Design review of the part built by this model. Coordinates are the model's own, in mm. A direction names the side the tool comes from. Coordinates: 2 decimals unless noted, no trailing zeros. Write each loop counter-clockwise with the first axis right and the second up, starting at its lowest first coordinate (ties: lowest second). Pieces come first, ordered by that corner, then holes. Notation, with made-up numbers: (-24.5, -22.75) - (0.5, -22.75) arc R9 ccw to (0.5, -8.75) - close; hole circle Ø1 at (75.5, 23). An arc over 180 degrees is marked (long way). Use a Markdown table: item, result.
from build123d import *

# Parameters (mm, degrees)
F3_DEPTH = 50
F4_DEPTH = 50
F5_DEPTH = 50


with BuildPart() as f3:
    # F0 (on Top) → F3 (new body, symmetric)
    with BuildSketch(Plane.XY):
        Polygon((50, -27.040666), (50, 50), (25.545932, 50), (25.545932, -27.040666), (-25.926208, -27.040666), (-25.926208, -8.301959), (-50, -8.301959), (-50, -27.040666), (-50, -50), (-25.926208, -50), (25.545932, -50), (50, -50), align=None)
    extrude(amount=F3_DEPTH, both=True)

    # F1 (on Front) → F4 (intersect, symmetric)
    with BuildSketch(Plane.XZ):
        Polygon((-29.175453, 50), (-50, 50), (-50, -50), (-29.175453, -50), (-29.175453, 20.161899), (-12.334338, -50), (12.334337, -50), (28.463857, 28.938254), (28.463857, -50), (50, -50), (50, 50), (28.463857, 50), (12.334337, -10.199549), (12.334337, 50), (-12.334338, 50), (-12.334338, -10.436747), align=None)
    extrude(amount=F4_DEPTH, both=True, mode=Mode.INTERSECT)

    # F2 (on Right) → F5 (intersect, symmetric)
    with BuildSketch(Plane.YZ):
        Polygon((-26.566265, 50), (-50, 50), (-50, -50), (-26.566265, -50), (-26.566265, 27.98946), (-9.725152, -50), (11.148345, -50), (27.752262, 25.617471), (27.752262, -50), (50, -50), (50, 50), (27.752262, 50), (11.148345, -11.385542), (11.148345, 50), (-9.725152, 50), (-9.725152, -12.334338), align=None)
    extrude(amount=F5_DEPTH, both=True, mode=Mode.INTERSECT)


solid = f3.part
(1) For pin 1 (8 mm diameter, centred on x = -33, z = 31, fed in from +Y); pin 2 (10.5 mm diameter, centred on y = 5.5, z = 27, fed in from -X); pin 3 (0.7 mm diameter, centred on x = 27, z = 18.5, fed in from -Y), all flat-tipped, find the tip position at first contact; note any pin that passes through.
Determined:
| item | result |
|---|---|
| pin 1 | y = -8.3 |
| pin 2 | x = 25.55 |
| pin 3 | through |
(2) Draft analysis for pull direction Y (two halves, no side actions). For faces 1 (the flat face through (26.322, -25.787, 24.38)), 2 (the flat face through (-38, -8.302, 1)), 3 (the flat face through (25.546, 1, 27)), state which applies: +Y half, -Y half, draft (parallel to the pull), parting line (faces both ways), or undercut.
Determined:
| item | result |
|---|---|
| face 1 | undercut |
| face 2 | +Y half |
| face 3 | draft |
(3) For L1, parallel to Y at x = 40, z = -18.5; L2, parallel to X at y = -31, z = -41.5; L3, parallel to Y at x = 34.5, z = 10, list the stretches that pass through material, from the lowest coordinate up. Write a range as from..to.
Determined:
| item | result |
|---|---|
| L1 | -50..-26.57, -16.53..18.07, 27.75..50 |
| L2 | -50..-29.18, -14.37..14.07, 28.46..50 |
| L3 | -50..-26.57, -22.68..-15.76, -9.73..11.15, 16.93..24.32, 27.75..50 |
(4) Take a section at B-B on z = -25.5. Write out the cut boundary in (x, y), and give its area (3 significant figures).
Determined:
| item | result |
|---|---|
| outline | (-50, -50) - (-29.18, -50) - (-29.18, -26.57) - (-50, -26.57) - close; (-50, -15.02) - (-29.18, -15.02) - (-29.18, -8.3) - (-50, -8.3) - close; (-18.22, -50) - (17.34, -50) - (17.34, -27.04) - (-18.22, -27.04) - close; (28.46, -50) - (50, -50) - (50, -26.57) - (28.46, -26.57) - close; (28.46, -15.02) - (50, -15.02) - (50, 16.53) - (28.46, 16.53) - close; (28.46, 27.75) - (50, 27.75) - (50, 50) - (28.46, 50) - close |
| area | 3,110 mm2 |
(5) Take a section at C-C on x = 40.5. Write out the cut boundary in (y, z), and give its area (3 significant figures).
Determined:
| item | result |
|---|---|
| outline | (-50, -50) - (-26.57, -50) - (-26.57, 27.99) - (-9.73, -50) - (11.15, -50) - (27.75, 25.62) - (27.75, -50) - (50, -50) - (50, 50) - (27.75, 50) - (11.15, -11.39) - (11.15, 50) - (-9.73, 50) - (-9.73, -12.33) - (-26.57, 50) - (-50, 50) - close |
| area | 7,680 mm2 |
(6) Take a section at A-A on y = 36. Write out the cut boundary in (x, z).
Determined:
| item | result |
|---|---|
| outline | (25.55, 14.66) - (28.46, 28.94) - (28.46, -50) - (50, -50) - (50, 50) - (28.46, 50) - (25.55, 39.11) - close |
(7) Machinability: for faces 4 (the flat face through (0, -27.041, 1)), 5 (the flat face through (-50, -33, 1)), 6 (the flat face through (-27.53, -9.02, 44.09)), 7 (the flat face through (39.383, -18.264, -10.459)), which of the approach directions +Z, -Z, +X, -X, +Y, -Y give a long, thin tool a straight path to every point of the face, cutting with its end or side? Answer none if there is none.
Determined:
| item | result |
|---|---|
| face 4 | +Z, -Z, +Y |
| face 5 | +Z, -Z, -X, +Y, -Y |
| face 6 | +Z, +Y, -Y |
| face 7 | -Z, +X, -X |
(8) Take a section at D-D on y = -12.5. Write out the cut boundary in (x, z).
Determined:
| item | result |
|---|---|
| outline | (-50, -37.15) - (-29.18, -37.15) - (-29.18, -2.06) - (-50, -2.06) - close; (28.46, -37.15) - (50, -37.15) - (50, -2.06) - (28.46, -2.06) - close |
